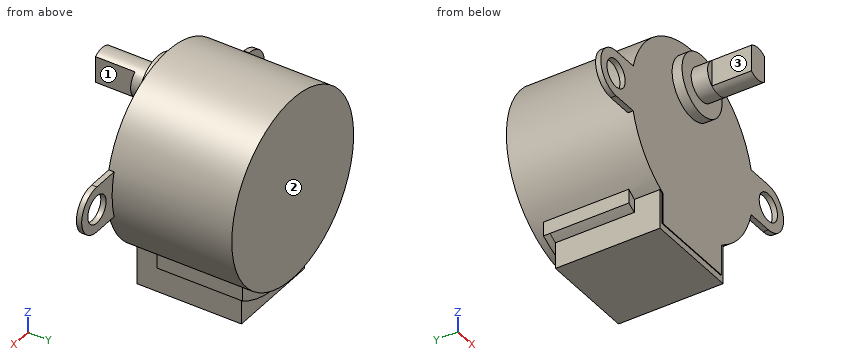
from build123d import *

# Parameters (mm, degrees)
SKETCH010_R     = 14
PAD005_DEPTH    = 19
SKETCH011_W     = 14.5
SKETCH011_H     = 6.02346
PAD006_DEPTH    = 16
SKETCH012_R     = 2.1
PAD007_DEPTH    = 0.8
SKETCH013_R     = 4.6
PAD008_DEPTH    = 1.5
SKETCH014_R     = 2.5
PAD009_DEPTH    = 2.5
PAD010_DEPTH    = 6
PAD011_DEPTH    = 12
PAD012_DEPTH    = 1
POCKET006_DEPTH = 0.1


with BuildPart() as part:
    # Sketch010 → Pad005 (new body)
    with BuildSketch(Plane.XZ):
        Circle(SKETCH010_R)
    extrude(amount=-PAD005_DEPTH)

    # Sketch011 (on Face2 of Pad005) → Pad006 (join)
    with BuildSketch(Plane.XZ):
        with Locations((0, -14.98827)):
            Rectangle(SKETCH011_W, SKETCH011_H)
    extrude(amount=-PAD006_DEPTH)

    # Sketch012 (on Face7 of Pad006) → Pad007 (join)
    with BuildSketch(Plane.XZ):
        with BuildLine():
            ThreePointArc((-17.5, 3.5), (-21, 0), (-17.5, -3.5))
            Line((-13.555442, -3.5), (-17.5, -3.5))
            Line((-13.555442, 3.5), (-13.555442, -3.5))
            Line((-17.5, 3.5), (-13.555442, 3.5))
        make_face()
        with Locations((-17.5, 0)):
            Circle(SKETCH012_R, mode=Mode.SUBTRACT)
    pad007 = extrude(amount=-PAD007_DEPTH)

    # Mirrored: Pad007 across Sketch012 V_Axis
    add(pad007.mirror(Plane(origin=(0, 0, 0), x_dir=(0, -1, 0), z_dir=(1, 0, 0))))

    # Sketch013 (on Face17 of Mirrored) → Pad008 (join)
    with BuildSketch(Plane.XZ):
        with Locations((0, 8)):
            Circle(SKETCH013_R)
    extrude(amount=PAD008_DEPTH)

    # Sketch014 (on Face19 of Pad008) → Pad009 (join)
    with BuildSketch(Plane.XZ.offset(1.5)):
        with Locations((0, 8)):
            Circle(SKETCH014_R)
    extrude(amount=PAD009_DEPTH)

    # Sketch015 (on Face21 of Pad009) → Pad010 (join)
    with BuildSketch(Plane.XZ.offset(4)):
        with BuildLine():
            Line((-1.5, 10), (-1.5, 6))
            ThreePointArc((-1.5, 6), (0, 5.5), (1.5, 6))
            Line((1.5, 10), (1.5, 6))
            ThreePointArc((1.5, 10), (0, 10.5), (-1.5, 10))
        make_face()
    extrude(amount=PAD010_DEPTH)

    # Sketch016 (on DatumPlane) → Pad011 (join)
    with BuildSketch(Plane.XZ.offset(-4)):
        with BuildLine():
            ThreePointArc((-8.5, -13.278272), (-7.883264, -13.653448), (-7.25, -14))
            Line((-7.25, -14), (-7.25, -11.97654))
            ThreePointArc((-8.5, -11.124298), (-7.88652, -11.567316), (-7.25, -11.97654))
            Line((-8.5, -13.278272), (-8.5, -11.124298))
        make_face()
    pad011 = extrude(amount=-PAD011_DEPTH)

    # Mirrored001: Pad011 across Sketch016 V_Axis
    add(pad011.mirror(Plane(origin=(0, 4, 0), x_dir=(0, -1, 0), z_dir=(1, 0, 0))))

    # Sketch017 (on Face31 of Mirrored001) → Pad012 (join)
    with BuildSketch(Plane(origin=(0, 16, 0), x_dir=(1, 0, 0), z_dir=(0, 1, 0))):
        with BuildLine():
            ThreePointArc((8.5, 11.124298), (0, 14), (-8.5, 11.124298))
            Line((-8.5, 13.278272), (-8.5, 11.124298))
            ThreePointArc((8.5, 13.278272), (0, 15.765865), (-8.5, 13.278272))
            Line((8.5, 13.278272), (8.5, 11.124298))
        make_face()
    extrude(amount=PAD012_DEPTH)

    # Sketch018 (on Face9 of Pad012) → Pocket006 (cut)
    with BuildSketch(Plane.XZ):
        with BuildLine():
            Line((-7.25, -11.97654), (-7.25, -18))
            Line((7.25, -18), (-7.25, -18))
            Line((7.25, -18), (7.25, -11.97654))
            ThreePointArc((6.75, -12.265297), (7.001278, -12.123131), (7.25, -11.97654))
            Line((6.75, -17), (6.75, -12.265297))
            Line((-6.75, -17), (6.75, -17))
            Line((-6.75, -12.265297), (-6.75, -17))
            ThreePointArc((-7.25, -11.97654), (-7.001489, -12.123496), (-6.75, -12.265297))
        make_face()
    extrude(amount=-POCKET006_DEPTH, mode=Mode.SUBTRACT)


solid = part.part
Geometry check sheet. Reference: the model listing, model coordinates, mm. Face numbers are marked on the shaded views. A direction names the side the tool comes from. Round coordinates to 2 decimals unless told otherwise and drop trailing zeros. Order: outer loops, then holes, each group sorted by start corner. A loop starts at its lowest first (then second) coordinate and runs counter-clockwise, first axis right, second up. Notation, with made-up numbers: M 0,5.25 L 13,5.25 A20 cw 13,9.25 Z; hole C 43.5,3 d1. An arc over 180 degrees is marked long. Write each question's results on one line, items separated by ' | '. Start each with the question number.
1. Go/stop test with flat-tipped pins: P1, Ø3.5, axis at x = 16, z = 1.5, coming from the +Y side; P2, Ø3, axis at x = -2.5, y = 1, coming from the +Z side; P3, Ø3, axis at y = 8, z = -15, coming from the -X side; P4, Ø6, axis at y = -4.5, z = -5, coming from the +X side (3 decimals). Record where each tip stops, or that it passes through.
2. Cross-section at C-C on y = 11.75. Record the boundary of the cut face in (x, z).
3. Cross-section at D-D on z = 8. Record the boundary of the cut face in (x, y), plus the area to 3 significant figures.
4. Cross-section at A-A on z = 0. Record the boundary of the cut face in (x, y), plus the area to 3 significant figures.
5. Set-up check for the marked faces 1, 2 and 3: record each of +Z, -Z, +X, -X, +Y, -Y from which the full face is reachable in a straight line by a thin tool's end or side.
6. Cross-section at B-B on x = 0. Record the boundary of the cut face in (y, z), plus the area to 3 significant figures.
7. Material ranges on L1, parallel to Z at x = -17.5, y = 0.4; L2, parallel to Y at x = 5, z = 3.5; L3, parallel to X at y = 2, z = -12.5, recorded low to high. Write a range as from..to.
Resolved:
1) P1: y = 0.8 | P2: z = 13.96 | P3: x = -8.14 | P4: through
2) outline: M -8.5,-13.28 A15.77 ccw -7.25,-14 L -7.25,-18 L 7.25,-18 L 7.25,-14 A15.77 ccw 8.5,-13.28 L 8.5,-11.12 A14 ccw long -8.5,-11.12 Z
3) outline: M -11.49,0 L -4.6,0 L -4.6,-1.5 L -2.5,-1.5 L -2.5,-4 L -1.5,-4 L -1.5,-10 L 1.5,-10 L 1.5,-4 L 2.5,-4 L 2.5,-1.5 L 4.6,-1.5 L 4.6,0 L 11.49,0 L 11.49,19 L -11.49,19 Z | area: 481 mm2
4) outline: M -21,0 L -19.6,0 L -19.6,0.8 L -21,0.8 Z; M -15.4,0 L 15.4,0 L 15.4,0.8 L 14,0.8 L 14,19 L -14,19 L -14,0.8 L -15.4,0.8 Z; M 19.6,0 L 21,0 L 21,0.8 L 19.6,0.8 Z | area: 536 mm2
5) face 1: +Z, -Z, +X, -Y | face 2: +Z, -Z, +X, -X, +Y | face 3: +Z, -Z, -X, -Y
6) outline: M -10,5.5 L -1.5,5.5 L -1.5,3.4 L 0,3.4 L 0,-17 L 0.1,-17 L 0.1,-18 L 16,-18 L 16,-15.77 L 17,-15.77 L 17,-14 L 19,-14 L 19,14 L 0,14 L 0,12.6 L -1.5,12.6 L -1.5,10.5 L -10,10.5 Z | area: 654 mm2
7) L1: -3.5..-2.1, 2.1..3.5 | L2: 0..19 | L3: -7.25..7.25
